```python
from build123d import *

# Parameters (mm, degrees)
F1_DEPTH = 22
F2_DEPTH = 5
F3_DEPTH = 5
F4_DEPTH = 3


with BuildPart() as f1:
    # F0 (on Front) → F1 (new body)
    with BuildSketch(Plane.XZ):
        with BuildLine():
            Line((4.5, 24.591665), (4.5, 25.099801))
            ThreePointArc((4.5, 25.099801), (3.129623, 25.307222), (1.75, 25.43988))
            Line((1.75, 25.43988), (1.75, 21.921448))
            Line((1.75, 21.921448), (2, 21.921448))
            Line((2, 21.921448), (5.499875, 21.921448))
            Line((5.499875, 21.921448), (5.499875, 17.421448))
            Line((5.499875, 17.421448), (0, 17.421448))
            Line((0, 17.421448), (-5.499875, 17.421448))
            Line((-5.499875, 17.421448), (-5.499875, 21.921448))
            Line((-5.499875, 21.921448), (-2, 21.921448))
            Line((-2, 21.921448), (-1.75, 21.921448))
            Line((-1.75, 21.921448), (-1.75, 25.43988))
            ThreePointArc((-1.75, 25.43988), (-3.129623, 25.307222), (-4.5, 25.099801))
            Line((-4.5, 25.099801), (-4.5, 24.591665))
            ThreePointArc((-4.5, 24.591665), (-5.757605, 24.327967), (-7, 24))
            Line((-7, 24), (-7, 15))
            Line((-7, 15), (0, 15))
            Line((0, 15), (7, 15))
            Line((7, 15), (7, 24))
            ThreePointArc((7, 24), (5.757605, 24.327967), (4.5, 24.591665))
        make_face()
    extrude(amount=F1_DEPTH)

    # F0 (on Front) → F2 (join)
    with BuildSketch(Plane.XZ):
        with BuildLine():
            Line((-4.5, 24.591665), (-4.5, 25.099801))
            ThreePointArc((-4.5, 25.099801), (-5.757293, 24.841569), (-7, 24.5204))
            Line((-7, 24.5204), (-7, 24))
            ThreePointArc((-7, 24), (-5.757605, 24.327967), (-4.5, 24.591665))
        make_face()
    extrude(amount=F2_DEPTH)

    # F0 (on Front) → F3 (join)
    with BuildSketch(Plane.XZ):
        with BuildLine():
            Line((7, 24), (7, 24.5204))
            ThreePointArc((7, 24.5204), (5.757293, 24.841569), (4.5, 25.099801))
            Line((4.5, 25.099801), (4.5, 24.591665))
            ThreePointArc((4.5, 24.591665), (5.757605, 24.327967), (7, 24))
        make_face()
    extrude(amount=F3_DEPTH)

    # F0 (on Front) → F4 (join)
    with BuildSketch(Plane.XZ):
        with BuildLine():
            Line((1.75, 21.921448), (1.75, 25.43988))
            ThreePointArc((1.75, 25.43988), (0, 25.5), (-1.75, 25.43988))
            Line((-1.75, 25.43988), (-1.75, 21.921448))
            Line((-1.75, 21.921448), (-2, 21.921448))
            Line((-2, 21.921448), (-5.499875, 21.921448))
            Line((-5.499875, 21.921448), (-5.499875, 17.421448))
            Line((-5.499875, 17.421448), (0, 17.421448))
            Line((0, 17.421448), (5.499875, 17.421448))
            Line((5.499875, 17.421448), (5.499875, 21.921448))
            Line((5.499875, 21.921448), (2, 21.921448))
            Line((2, 21.921448), (1.75, 21.921448))
        make_face()
    extrude(amount=F4_DEPTH)


solid = f1.part
```
Geometry: final body of the model. Coordinates: model frame, mm. A direction names the side the tool comes from. Coordinates: 2 decimals unless noted, no trailing zeros. Order: outer loops, then holes, each group sorted by start corner. A loop starts at its lowest first (then second) coordinate and runs counter-clockwise, first axis right, second up. Notation, with made-up numbers: (79, 51) -> (115, 51) arc R20 ccw to (115, 55) -> close; hole circle Ø6 at (26, -18). An arc over 180 degrees is marked (long way). Write item = value, one per line.
(1) Cut plane D-D on z = 24.25. Return loops of the section in (x, y), plus the area to 3 significant figures.
Solved:
outline = (-7, -5) -> (-6.08, -5) -> (-6.08, -22) -> (-1.75, -22) -> (-1.75, -3) -> (1.75, -3) -> (1.75, -22) -> (6.08, -22) -> (6.08, -5) -> (7, -5) -> (7, 0) -> (-7, 0) -> close
area = 210 mm²
(2) Cut plane A-A on z = 18.75. Return loops of the section in (x, y).
Solved:
outline = (-7, -22) -> (-5.5, -22) -> (-5.5, -3) -> (5.5, -3) -> (5.5, -22) -> (7, -22) -> (7, 0) -> (-7, 0) -> close
(3) Cut plane B-B on y = -14.5. Return loops of the section in (x, z), plus the area to 3 significant figures.
Solved:
outline = (-7, 15) -> (7, 15) -> (7, 24) arc R25 ccw to (4.5, 24.59) -> (4.5, 25.1) arc R25.5 ccw to (1.75, 25.44) -> (1.75, 21.92) -> (5.5, 21.92) -> (5.5, 17.42) -> (-5.5, 17.42) -> (-5.5, 21.92) -> (-1.75, 21.92) -> (-1.75, 25.44) arc R25.5 ccw to (-4.5, 25.1) -> (-4.5, 24.59) arc R25 ccw to (-7, 24) -> close
area = 77.9 mm²
(4) Line query: line 1 (X direction, y = -13, z = 22); line 2 (X direction, y = -12.75, z = 25); line 3 (Y direction, x = 1.75, z = 21.75). Output: solid intervals per line, ascending.
Solved:
line_1 = -7 to -1.75, 1.75 to 7
line_2 = -4.5 to -1.75, 1.75 to 4.5
line_3 = -3 to 0
(5) Cut plane C-C on x = 2.5. Return loops of the section in (y, z).
Solved:
outline = (-22, 15) -> (0, 15) -> (0, 25.38) -> (-22, 25.38) -> (-22, 21.92) -> (-3, 21.92) -> (-3, 17.42) -> (-22, 17.42) -> close
(6) Pull-direction query (Z, two-part tool) for faces 6 (the flat face through (4, -12, 21.921)), 7 (the flat face through (1.75, -12, 24)), 8 (the cylindrical face through (5.775, -13.381, 24.324)); classes: pulls with the +Z half, pulls with the -Z half, needs draft (parallel to the pull), parting line crosses it, or undercut.
Solved:
face_6 = undercut
face_7 = needs draft
face_8 = pulls with the +Z half
(7) Pin query (flat end, axial travel): pin 1 Ø3 at (x, z) = (1.5, 19) entering from -Y; pin 2 Ø6 at (x, y) = (2, -7) entering from +Z; pin 3 Ø6 at (x, y) = (0, -5.5) entering from +Z; pin 4 Ø0.9 at (x, z) = (5, 25) entering from -Y. Return the tip coordinate at first contact, or that it passes through.
Solved:
pin_1 = -3
pin_2 = 25.44
pin_3 = 25.5
pin_4 = -5
(8) Access query for faces 1 (the flat face through (-1.75, -12, 24)), 2 (the flat face through (-5.5, -12, 20)), 3 (the flat face through (-7, -11, 20)), 4 (the flat face through (5.7, -5, 24.6)), 5 (the flat face through (-5.8, -5, 24.6)). Directions: +Z, -Z, +X, -X, +Y, -Y. A direction counts if a zero-diameter tool reaches every point of the face in a straight line with its end or side. Return the directions, or none.
Solved:
face_1 = +Z, -Y
face_2 = -Y
face_3 = +Z, -Z, -X, +Y, -Y
face_4 = +Z, +X, -Y
face_5 = +Z, -X, -Y
